Could you check a few things on this model? Use its own coordinates, in mm. Face numbers are marked on the shaded views. Give positions to 0.01 mm unless a question says otherwise; leave off trailing zeros. Loops run counter-clockwise (first coordinate to the right, second up) from the corner with the lowest first, then second, coordinate; pieces in that order, holes last. Notation, with made-up numbers: (69, 52.25) - (103, 52.25) arc R33 ccw to (103, 85.25) - close; hole circle Ø8 at (-36.5, -13.75). An arc over 180 degrees is marked (long way). Write each question's results on one line, items separated by ' | '. Start each with the question number.
1) If we mould it in two halves opening along Y, with no side actions, what happens to the marked faces 1, 2 and 3? For each: +Y half, -Y half, draft (parallel to the pull), parting line (faces both ways), or undercut.
2) I'm going to push flat-ended pins straight in: pin 1 (6 mm diameter, centred on x = 52, y = 19, fed in from -Z); pin 2 (5 mm diameter, centred on y = 23.5, z = -42.5, fed in from -X); pin 3 (5 mm diameter, centred on y = 18, z = 34, fed in from +X). Where does each tip first touch, or does it pass through?
3) I want a section at A-A, the plane x = 0. Write out the boundary of the cut face in (y, z) (1 decimal).
4) If I drill on probe 1 along X at (y, z) = (18.5, 0) (1 decimal); probe 2 along Y at (x, z) = (-25, -6.5) (3 decimals); probe 3 along Z at (x, y) = (-13, 13), over which ranges is the centre line in solid material (lowest first)? Write a range as [from, to].
5) I want a section at B-B, the plane z = 0. Write out the boundary of the cut face in (x, y) (1 decimal), and give its area (3 significant figures).
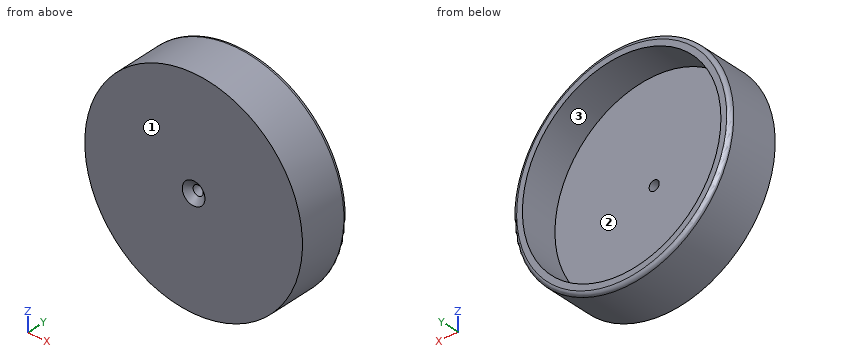
from build123d import *

# Parameters (mm, degrees)
SKETCH1_R                                           = 73.025
BOSS_EXTRUDE1_DEPTH                                 = 9.525
SKETCH2_R                                           = 73.025
SKETCH2_R_2                                         = 66.6115
BOSS_EXTRUDE2_DEPTH                                 = 25.4
CSK_FOR_1_4_FLAT_HEAD_MACHINE_SCREW_100_D           = 6.7564
CSK_FOR_1_4_FLAT_HEAD_MACHINE_SCREW_100_DEPTH       = 10.16
CSK_FOR_1_4_FLAT_HEAD_MACHINE_SCREW_100_CSINK_D     = 15.24
CSK_FOR_1_4_FLAT_HEAD_MACHINE_SCREW_100_CSINK_ANGLE = 100
CSK_FOR_1_4_FLAT_HEAD_MACHINE_SCREW_100_TIP         = 2.029827343
FILLET1_R                                           = 2.54


with BuildPart() as part:
    # Sketch1 → Boss-Extrude1 (new body)
    with BuildSketch(Plane(origin=(0, 0, 0), x_dir=(1, 0, 0), z_dir=(0, 1, 0))):
        with Locations(Location((0, 0, 0), (0, 0, 90))):
            Circle(SKETCH1_R)
    extrude(amount=BOSS_EXTRUDE1_DEPTH)

    # Sketch2 → Boss-Extrude2 (add)
    with BuildSketch(Plane(origin=(0, 9.525, 0), x_dir=(1, 0, 0), z_dir=(0, 1, 0))):
        with Locations(Location((0, 0, 0), (0, 0, 90))):
            Circle(SKETCH2_R)
        with Locations(Location((0, 0, 0), (0, 0, 270))):
            Circle(SKETCH2_R_2, mode=Mode.SUBTRACT)
    extrude(amount=BOSS_EXTRUDE2_DEPTH)

    # CSK for 1/4 Flat Head Machine Screw (100)1
    with Locations(Plane(origin=(0, 0, 0), x_dir=(-1, 0, 0), z_dir=(0, -1, 0))):
        with Locations((0, 0)):
            CounterSinkHole(CSK_FOR_1_4_FLAT_HEAD_MACHINE_SCREW_100_D / 2, CSK_FOR_1_4_FLAT_HEAD_MACHINE_SCREW_100_CSINK_D / 2, depth=CSK_FOR_1_4_FLAT_HEAD_MACHINE_SCREW_100_DEPTH, counter_sink_angle=CSK_FOR_1_4_FLAT_HEAD_MACHINE_SCREW_100_CSINK_ANGLE)
            with Locations((0, 0, -(CSK_FOR_1_4_FLAT_HEAD_MACHINE_SCREW_100_DEPTH + CSK_FOR_1_4_FLAT_HEAD_MACHINE_SCREW_100_TIP / 2))):  # 118° drill point
                Cone(0, CSK_FOR_1_4_FLAT_HEAD_MACHINE_SCREW_100_D / 2, CSK_FOR_1_4_FLAT_HEAD_MACHINE_SCREW_100_TIP, mode=Mode.SUBTRACT)

    # Fillet1
    fillet1_edges = [part.edges().sort_by_distance(p)[0] for p in [
        (0, 34.925, 73.025),
    ]]
    fillet(fillet1_edges, radius=FILLET1_R)


solid = part.part
Answers:
1) face 1: -Y half | face 2: +Y half | face 3: draft
2) pin 1: stops at z = -54.14 | pin 2: stops at x = -61.1 | pin 3: stops at x = 65.88
3) outline: (0, -73) - (32.4, -73) arc R2.5 ccw to (34.9, -70.5) - (34.9, -66.6) - (9.5, -66.6) - (9.5, -3.4) - (3.6, -3.4) - (0, -7.6) - close; (0, 7.6) - (3.6, 3.4) - (9.5, 3.4) - (9.5, 66.6) - (34.9, 66.6) - (34.9, 70.5) arc R2.5 ccw to (32.4, 73) - (0, 73) - close
4) probe 1: x = [-73, -66.6], [66.6, 73] | probe 2: y = [0, 9.525] | probe 3: z = [-71.86, -65.33], [65.33, 71.86]
5) outline: (-73, 0) - (-7.6, 0) - (-3.4, 3.6) - (-3.4, 9.5) - (-66.6, 9.5) - (-66.6, 34.9) - (-70.5, 34.9) arc R2.5 ccw to (-73, 32.4) - close; (3.4, 3.6) - (7.6, 0) - (73, 0) - (73, 32.4) arc R2.5 ccw to (70.5, 34.9) - (66.6, 34.9) - (66.6, 9.5) - (3.4, 9.5) - close | area: 1,630 mm2
